Could you check a few things on this drawing? It's one solid part, dimensions in mm from its lowest x, y, z. A direction names the side the tool comes from. Give positions to 0.01 mm unless a question says otherwise; leave off trailing zeros. Order: outer loops, then holes, each group sorted by start corner. A loop starts at its lowest first (then second) coordinate and runs counter-clockwise, first axis right, second up. Notation, with made-up numbers: (-26, 77.25) -> (-13, 77.25) arc R33 cw to (-13, 106.25) -> close; hole circle Ø11 at (32, 19.25). An arc over 180 degrees is marked (long way). Write each question's results on one line, items separated by ' | '. Start each with the question number.
Q1. I'm going to push flat-ended pins straight in: pin 1 (4.5 mm diameter, centred on y = 5.5, z = 25.5, fed in from -X); pin 2 (6.5 mm diameter, centred on x = 25, z = 10, fed in from +Y). Where does each tip first touch, or does it pass through?
Q2. Imagine slicing it at A-A, the plane x = 43. Please give me the cut outline in (y, z).
Q3. I need wall thicknesses on line 1 along Z through (x, y) = (7, 2.5); line 2 along Z through (x, y) = (5.5, 7.25); line 3 along X through (y, z) = (2.75, 20.5). Which ranges of each line are inside material? Lowest first, please. Write a range as [from, to].
Q4. For the marked faces 4, 5, 6, 7 and 8, which set-ups out of +Z, -Z, +X, -X, +Y, -Y let a thin tool reach every point of the face, with its end or its side?
Q5. Thinking about a two-plate mould opening in X: for the marked faces 1, 2 and 3, which applies, pulls with the +X half, pulls with the -X half, needs draft (parallel to the pull), parting line crosses it, or undercut?
Q6. Imagine slicing it at B-B, the plane z = 16.5. Please give me the cut outline in (x, y).
Q7. Imagine slicing it at C-C, the plane y = 4. Please give me the cut outline in (x, z), then the cut area to 3 significant figures.
Q8. Imagine slicing it at D-D, the plane x = 27.5. Please give me the cut outline in (y, z), then the cut area to 3 significant figures.
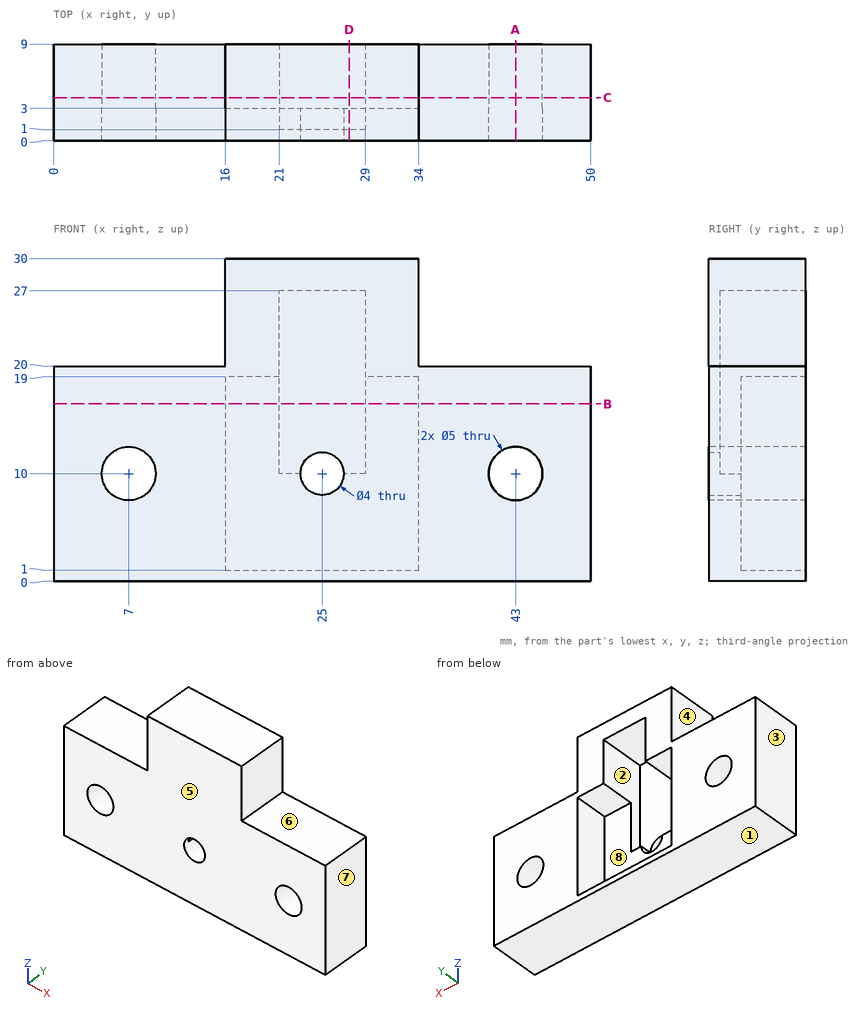
Geometry check:
1) pin 1: x = 16 | pin 2: y = 3
2) outline: (0, 0) -> (9, 0) -> (9, 7.5) -> (0, 7.5) -> close; (0, 12.5) -> (9, 12.5) -> (9, 20) -> (0, 20) -> close
3) line 1: [0, 7.5], [12.5, 20] | line 2: [0, 8], [12, 20] | line 3: [16, 21], [29, 34]
4) face 4: +Z, -X, +Y, -Y | face 5: +Z, -Z, +X, -X, -Y | face 6: +Z, +X, +Y, -Y | face 7: +Z, -Z, +X, +Y, -Y | face 8: +Y
5) face 1: needs draft | face 2: undercut | face 3: pulls with the -X half
6) outline: (0, 0) -> (50, 0) -> (50, 9) -> (34, 9) -> (34, 3) -> (29, 3) -> (29, 1) -> (21, 1) -> (21, 3) -> (16, 3) -> (16, 9) -> (0, 9) -> close
7) outline: (0, 0) -> (50, 0) -> (50, 20) -> (34, 20) -> (34, 30) -> (16, 30) -> (16, 20) -> (0, 20) -> close; hole circle Ø5 at (7, 10); hole (16, 1) -> (34, 1) -> (34, 19) -> (29, 19) -> (29, 27) -> (21, 27) -> (21, 19) -> (16, 19) -> close; hole circle Ø5 at (43, 10) | area: 753 mm²
8) outline: (0, 0) -> (9, 0) -> (9, 1) -> (3, 1) -> (3, 10) -> (1, 10) -> (1, 27) -> (9, 27) -> (9, 30) -> (0, 30) -> close | area: 80.0 mm²
